```python
from build123d import *

# Parameters (mm, degrees)
SKETCH1_R           = 3.683
BOSS_EXTRUDE1_DEPTH = 12.7
SKETCH2_R           = 3.683
BOSS_EXTRUDE2_DEPTH = 6.35


with BuildPart() as part:
    # Sketch1 → Boss-Extrude1 (new body)
    with BuildSketch(Plane.XY):
        with BuildLine():
            Line((97.79, -12.7), (-97.79, -12.7))
            ThreePointArc((-97.79, -12.7), (-100.484076836, -11.584076836), (-101.6, -8.89))
            Line((-101.6, -8.89), (-101.6, 8.89))
            ThreePointArc((-101.6, 8.89), (-100.484076836, 11.584076836), (-97.79, 12.7))
            Line((-97.79, 12.7), (97.79, 12.7))
            ThreePointArc((97.79, 12.7), (100.484076836, 11.584076836), (101.6, 8.89))
            Line((101.6, 8.89), (101.6, -8.89))
            ThreePointArc((101.6, -8.89), (100.484076836, -11.584076836), (97.79, -12.7))
        make_face()
        with Locations((-88.9, 0)):
            Circle(SKETCH1_R, mode=Mode.SUBTRACT)
        with Locations((88.9, 0)):
            Circle(SKETCH1_R, mode=Mode.SUBTRACT)
    extrude(amount=BOSS_EXTRUDE1_DEPTH)

    # Sketch2 → Boss-Extrude2 (add)
    with BuildSketch(Plane(origin=(0, 0, 0), x_dir=(-1, 0, 0), z_dir=(0, 0, -1))):
        with Locations((-88.9, 0)):
            Circle(SKETCH2_R)
        with Locations((88.9, 0)):
            Circle(SKETCH2_R)
    extrude(amount=-BOSS_EXTRUDE2_DEPTH)


solid = part.part
```
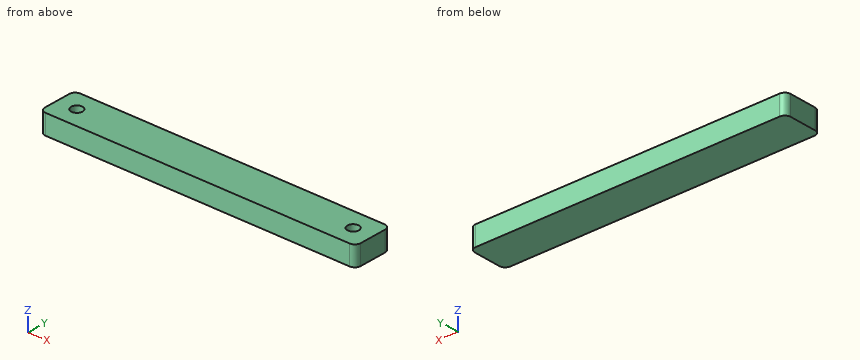
For this review, take the finished solid that the model builds, in its own axes (mm). Coordinates: 2 decimals unless noted, no trailing zeros. Order: outer loops, then holes, each group sorted by start corner. A loop starts at its lowest first (then second) coordinate and runs counter-clockwise, first axis right, second up. Notation, with made-up numbers: (-5.5, 43) - (34.5, 43) arc R11 ccw to (34.5, 48) - close; hole circle Ø11 at (65, -34). An arc over 180 degrees is marked (long way). Answer as a JSON object with one key per item and string values. Group by question number.
1. Clearance check with flat-ended pins moving along their axes: P1, Ø8.5, axis at x = 88.9, y = 0, coming from the +Z side; P2, Ø2, axis at x = 88.5, y = 1, coming from the +Z side. State where each tip first meets the part, or that it passes through.
2. For probe 1 along X at (y, z) = (0, 9.25); probe 2 along Y at (x, z) = (-88.9, 9.5); probe 3 along X at (y, z) = (-9, 7.5), list the stretches that pass through material, from the lowest coordinate up.
3. We need section A-A on z = 10.5. State the section outline as (x, y) points, then the cut area to 3 significant figures.
4. We need section C-C on y = 0. State the section outline as (x, z) points.
5. We need section B-B on x = -88.9. State the section outline as (y, z) points.
Final values:
{
 "1": {"P1": "z = 12.7", "P2": "z = 6.35"},
 "2": {"probe 1": "-101.6 to -92.58, -85.22 to 85.22, 92.58 to 101.6", "probe 2": "-12.7 to -3.68, 3.68 to 12.7", "probe 3": "-101.6 to 101.6"},
 "3": {"outline": "(-101.6, -8.89) arc R3.81 ccw to (-97.79, -12.7) - (97.79, -12.7) arc R3.81 ccw to (101.6, -8.89) - (101.6, 8.89) arc R3.81 ccw to (97.79, 12.7) - (-97.79, 12.7) arc R3.81 ccw to (-101.6, 8.89) - close; hole circle Ø7.37 at (-88.9, 0); hole circle Ø7.37 at (88.9, 0)", "area": "5,060 mm²"},
 "4": {"outline": "(-101.6, 0) - (101.6, 0) - (101.6, 12.7) - (92.58, 12.7) - (92.58, 6.35) - (85.22, 6.35) - (85.22, 12.7) - (-85.22, 12.7) - (-85.22, 6.35) - (-92.58, 6.35) - (-92.58, 12.7) - (-101.6, 12.7) - close"},
 "5": {"outline": "(-12.7, 0) - (12.7, 0) - (12.7, 12.7) - (3.68, 12.7) - (3.68, 6.35) - (-3.68, 6.35) - (-3.68, 12.7) - (-12.7, 12.7) - close"}
}
